from build123d import *

# Parameters (mm, degrees)
F0_W     = 73.396001
F0_H     = 108.268451
F1_DEPTH = 3.048
F2_R     = 15.275412
F3_DEPTH = 50.8
F4_R     = 4.02928
F5_DEPTH = 50.8


with BuildPart() as f1:
    # F0 (on Top) → F1 (new body)
    with BuildSketch(Plane.XY):
        with Locations((31.130662, 0.470406)):
            Rectangle(F0_W, F0_H)
    extrude(amount=F1_DEPTH)

    # F2 (on Front) → F3 (join)
    with BuildSketch(Plane.XZ):
        with Locations((-17.556151, 11.512231)):
            Circle(F2_R)
    extrude(amount=F3_DEPTH)

    # F4 (on face) → F5 (cut)
    with BuildSketch(Plane.XZ.offset(50.8)):
        with Locations((-17.556151, 11.512231)):
            Circle(F4_R)
    extrude(amount=-F5_DEPTH, mode=Mode.SUBTRACT)


solid = f1.part
Geometry check sheet. Reference: the model listing, model coordinates, mm. A direction names the side the tool comes from. Round coordinates to 2 decimals unless told otherwise and drop trailing zeros. Write each loop counter-clockwise with the first axis right and the second up, starting at its lowest first coordinate (ties: lowest second). Pieces come first, ordered by that corner, then holes.
Item 1: Section check C-C (x = 14). Record the boundary of the cut face in (y, z), plus the area to 3 significant figures.
Determined:
outline: (-53.66, 0) - (54.6, 0) - (54.6, 3.05) - (-53.66, 3.05) - close
area: 330 mm2
Item 2: Section check D-D (y = -6.5). Record the boundary of the cut face in (x, z).
Determined:
outline: (-5.57, 0) - (67.83, 0) - (67.83, 3.05) - (-4.84, 3.05) arc R15.28 ccw (long way) to (-5.57, 2.05) - close; hole circle Ø8.06 at (-17.56, 11.51)
Item 3: Section check A-A (z = 9). Record the boundary of the cut face in (x, y), plus the area to 3 significant figures.
Determined:
outline: (-32.62, -50.8) - (-20.71, -50.8) - (-20.71, 0) - (-32.62, 0) - close; (-14.41, -50.8) - (-2.49, -50.8) - (-2.49, 0) - (-14.41, 0) - close
area: 1,210 mm2
Item 4: Section check B-B (y = 41). Record the boundary of the cut face in (x, z), plus the area to 3 significant figures.
Determined:
outline: (-5.57, 0) - (67.83, 0) - (67.83, 3.05) - (-5.57, 3.05) - close
area: 224 mm2
Item 5: Access from +Z, -Z, +X, -X, +Y, -Y to the whole of each face (thin tool, end or side, straight path). Record for faces 1 (the face through (31, 1, 0)), 2 (the face through (31, -53.664, 2)).
Determined:
face 1: -Z, +X, +Y, -Y
face 2: +Z, -Z, +X, -X, -Y
Item 6: Go/stop test with flat-tipped pins: pin 1 Ø3 at (y, z) = (-22, 10.5) entering from +X; pin 2 Ø15.5 at (x, z) = (-18, 8.5) entering from -Y; pin 3 Ø6 at (y, z) = (28.5, 5) entering from +X; pin 4 Ø1.5 at (y, z) = (-15, 21) entering from +X. Record where each tip stops, or that it passes through.
Determined:
pin 1: stops at x = -2.28
pin 2: stops at y = -50.8
pin 3: stops at x = 67.83
pin 4: stops at x = -5.03
Item 7: Mould release check, pull along X, two halves, no side actions. Record for faces 3 (the face through (-5.567, 0, 1)), 4 (the face through (-21.58, -25.76, 11.69)), 5 (the face through (67.829, 0, 2)), 6 (the face through (-14, -50.8, 8)): +X half, -X half, draft (parallel to the pull), parting line (faces both ways), or undercut.
Determined:
face 3: undercut
face 4: undercut
face 5: +X half
face 6: draft
Item 8: Material ranges on line 1 along Z through (x, y) = (8, 34); line 2 along Y through (x, z) = (-27, 16); line 3 along X through (y, z) = (-41.5, 9.5), recorded low to high.
Determined:
line 1: z = 0 to 3.05
line 2: y = -50.8 to 0
line 3: x = -32.7 to -21.05, -14.07 to -2.41
